Job drawing, mm, ordinate dimensions from the low corner. One solid piece. Give positions to 0.01 mm unless a question says otherwise; leave off trailing zeros. Order: outer loops, then holes, each group sorted by start corner. A loop starts at its lowest first (then second) coordinate and runs counter-clockwise, first axis right, second up. Notation, with made-up numbers: M 46.5,47.5 L 78.5,47.5 A30 ccw 78.5,74.5 Z; hole C 5.25,-22 d4. An arc over 180 degrees is marked long. Use CSV: the item, a comma, the result in double quotes. Start each with the question number.
Item 1: Two-plate mould, pull along Z, no slides. Class the marked faces 1 and 2: pulls with the +Z half, pulls with the -Z half, needs draft (parallel to the pull), parting line crosses it, or undercut.
Item 2: Wall check: line 1 along X through (y, z) = (11, 136); line 2 along X through (y, z) = (9.25, 19). Give the ranges that are in metal, low to high.
Item 3: Band-saw the part on D-D on z = 94.5. Write the cut outline in (x, y), plus the area to 4 significant figures.
Item 4: Pin check, flat tips, straight feed: P1, Ø2, axis at y = 13, z = 97.5, coming from the +X side; P2, Ø2, axis at x = 95, z = 167, coming from the +Y side. Stop position of each tip, or through.
Item 5: Band-saw the part on C-C on y = 14.25. Give the number of separate pieces and of enclosed holes in the cut face, plus the area to 3 significant figures.
Item 6: Band-saw the part on B-B on x = 18. Write the cut outline in (y, z).
Item 7: Band-saw the part on A-A on z = 70.5. Write the cut outline in (x, y).
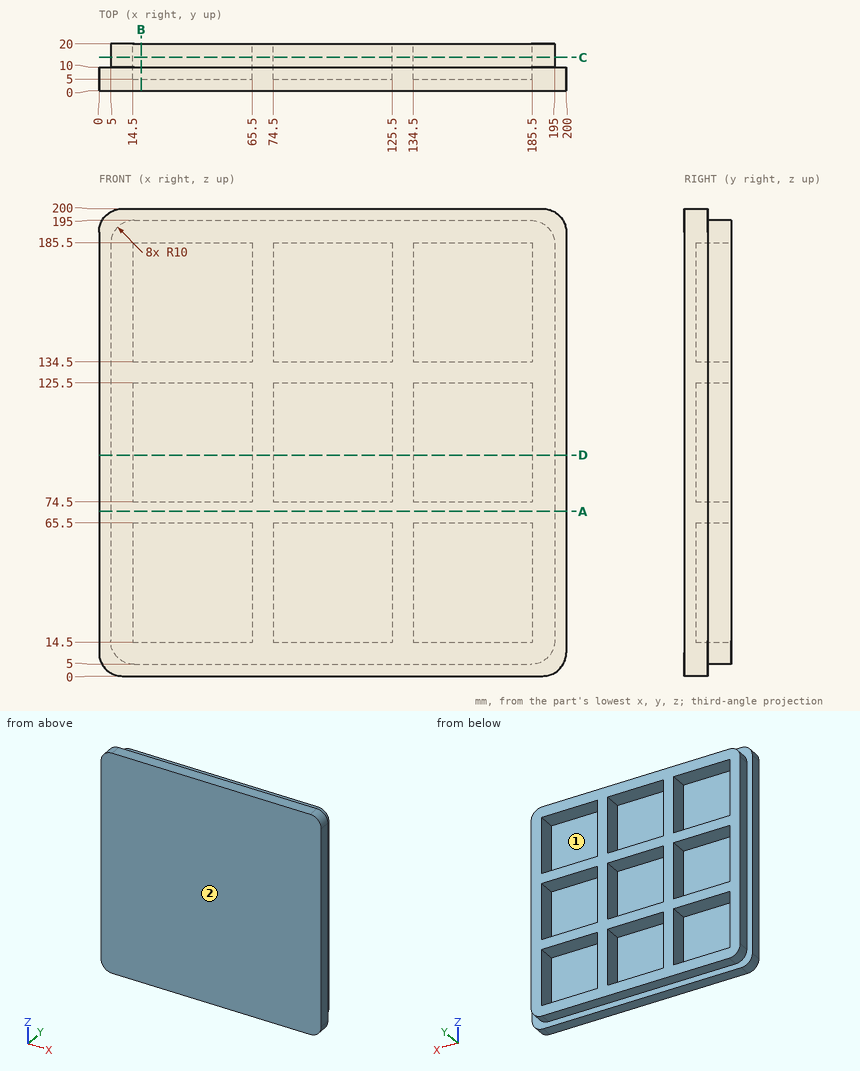
Model answer:
1,face 1,"undercut"
1,face 2,"needs draft"
2,line 1,"x = 5 to 14.5, 65.5 to 74.5, 125.5 to 134.5, 185.5 to 195"
2,line 2,"x = 0 to 14.5, 65.5 to 74.5, 125.5 to 134.5, 185.5 to 200"
3,outline,"M 0,0 L 200,0 L 200,10 L 195,10 L 195,20 L 185.5,20 L 185.5,5 L 134.5,5 L 134.5,20 L 125.5,20 L 125.5,5 L 74.5,5 L 74.5,20 L 65.5,20 L 65.5,5 L 14.5,5 L 14.5,20 L 5,20 L 5,10 L 0,10 Z"
3,area,"1,605 mm^2"
4,P1,"stops at x = 195"
4,P2,"stops at y = 5"
5,separate pieces,"1"
5,enclosed holes,"9"
5,area,"12,600 mm^2"
6,outline,"M 0,0 L 10,0 L 10,5 L 20,5 L 20,14.5 L 5,14.5 L 5,65.5 L 20,65.5 L 20,74.5 L 5,74.5 L 5,125.5 L 20,125.5 L 20,134.5 L 5,134.5 L 5,185.5 L 20,185.5 L 20,195 L 10,195 L 10,200 L 0,200 Z"
7,outline,"M 0,0 L 200,0 L 200,10 L 195,10 L 195,20 L 5,20 L 5,10 L 0,10 Z"
